Check sheet for the modelled part. Datum: model origin and axes. Units: mm. A direction names the side the tool comes from. Round coordinates to 2 decimals unless told otherwise and drop trailing zeros. Loops run counter-clockwise (first coordinate to the right, second up) from the corner with the lowest first, then second, coordinate; pieces in that order, holes last. Notation, with made-up numbers: (74.5, 83.25) - (90.5, 83.25) arc R28 cw to (90.5, 103.25) - close; hole circle Ø9 at (-26.5, 16.5). An arc over 180 degrees is marked (long way). Put each result on its own line as item: value. Start each with the question number.
Item 1: Section check D-D, the plane x = 12.75. Record the cut outline in (y, z).
Item 2: Draft check along Y on faces 4 (the flat face through (0, 9, 2)), 5 (the flat face through (-12.25, 0, 3)), 6 (the flat face through (0, 8, 0)), 7 (the flat face through (0, -9, 2)). Enter one of: pulls with the +Y half, pulls with the -Y half, needs draft (parallel to the pull), parting line crosses it, or undercut.
Item 3: Section check C-C, the plane y = 2. Record the cut outline in (x, z).
Item 4: Section check A-A, the plane x = 6.5. Record the cut outline in (y, z), and give its area (3 significant figures).
Item 5: Section check B-B, the plane z = 3. Record the cut outline in (x, y).
Item 6: Material ranges on line 1 along X through (y, z) = (-4.5, 3.9); line 2 along Y through (x, z) = (-7.5, 2.5); line 3 along X through (y, z) = (-5.25, 0.4), recorded low to high.
Item 7: Tool access check on faces 1 (the flat face through (-13, -7, 3)), 2 (the flat face through (-1, 7, 5)), 3 (the flat face through (0, 6, 2)). Record the directions out of +Z, -Z, +X, -X, +Y, -Y that give a thin tool (end or side, any length) a straight path to the whole face; none if there is none.
Item 8: Gauge pin test, flat ends, axial feed: pin 1 Ø1.6 at (x, y) = (-13, -2.5) entering from +Z; pin 2 Ø0.6 at (x, y) = (13.5, 2) entering from +Z. Record the tip position at first contact, or that the pin passes through.
from build123d import *

# Parameters (mm, degrees)
SKETCH1_W           = 30
SKETCH1_H           = 18
SKETCH1_W_2         = 22.5
SKETCH1_H_2         = 12
BOSS_EXTRUDE2_DEPTH = 5
SKETCH2_W           = 2
SKETCH2_H           = 14
SKETCH2_H_2         = 14.02224411
CUT_EXTRUDE1_DEPTH  = 4


with BuildPart() as part:
    # Sketch1 → Boss-Extrude2 (new body)
    with BuildSketch(Plane.XY):
        Rectangle(SKETCH1_W, SKETCH1_H)
        Rectangle(SKETCH1_W_2, SKETCH1_H_2, mode=Mode.SUBTRACT)
    extrude(amount=BOSS_EXTRUDE2_DEPTH)

    # Sketch2 → Cut-Extrude1 (cut)
    with BuildSketch(Plane.XY.offset(5)):
        with Locations((-13.25, 0)):
            Rectangle(SKETCH2_W, SKETCH2_H)
        with Locations((13.25, 0.011122055)):
            Rectangle(SKETCH2_W, SKETCH2_H_2)
    extrude(amount=-CUT_EXTRUDE1_DEPTH, mode=Mode.SUBTRACT)


solid = part.part
Check result:
1. outline: (-9, 0) - (9, 0) - (9, 5) - (7.02, 5) - (7.02, 1) - (-7, 1) - (-7, 5) - (-9, 5) - close
2. face 4: pulls with the +Y half
2. face 5: undercut
2. face 6: needs draft
2. face 7: pulls with the -Y half
3. outline: (-15, 0) - (-11.25, 0) - (-11.25, 5) - (-12.25, 5) - (-12.25, 1) - (-14.25, 1) - (-14.25, 5) - (-15, 5) - close; (11.25, 0) - (15, 0) - (15, 5) - (14.25, 5) - (14.25, 1) - (12.25, 1) - (12.25, 5) - (11.25, 5) - close
4. outline: (-9, 0) - (-6, 0) - (-6, 5) - (-9, 5) - close; (6, 0) - (9, 0) - (9, 5) - (6, 5) - close
4. area: 30.0 mm²
5. outline: (-15, -9) - (15, -9) - (15, 9) - (-15, 9) - close; hole (-14.25, -7) - (-12.25, -7) - (-12.25, 7) - (-14.25, 7) - close; hole (-11.25, -6) - (11.25, -6) - (11.25, 6) - (-11.25, 6) - close; hole (12.25, -7) - (14.25, -7) - (14.25, 7.02) - (12.25, 7.02) - close
6. line 1: -15 to -14.25, -12.25 to -11.25, 11.25 to 12.25, 14.25 to 15
6. line 2: -9 to -6, 6 to 9
6. line 3: -15 to -11.25, 11.25 to 15
7. face 1: +Z
7. face 2: +Z, +X, -X, +Y, -Y
7. face 3: +Z, -Z
8. pin 1: z = 5
8. pin 2: z = 1
